Job drawing, mm, ordinate dimensions from the low corner. One solid piece. A direction names the side the tool comes from. Round coordinates to 2 decimals unless told otherwise and drop trailing zeros. Order: outer loops, then holes, each group sorted by start corner. A loop starts at its lowest first (then second) coordinate and runs counter-clockwise, first axis right, second up. Notation, with made-up numbers: (58.25, -4) - (83.25, -4) arc R10 ccw to (83.25, 1) - close; hole circle Ø9 at (-37.75, 28.5). An arc over 180 degrees is marked (long way). Write each question's results on one line, items separated by ' | '. Start each with the question number.
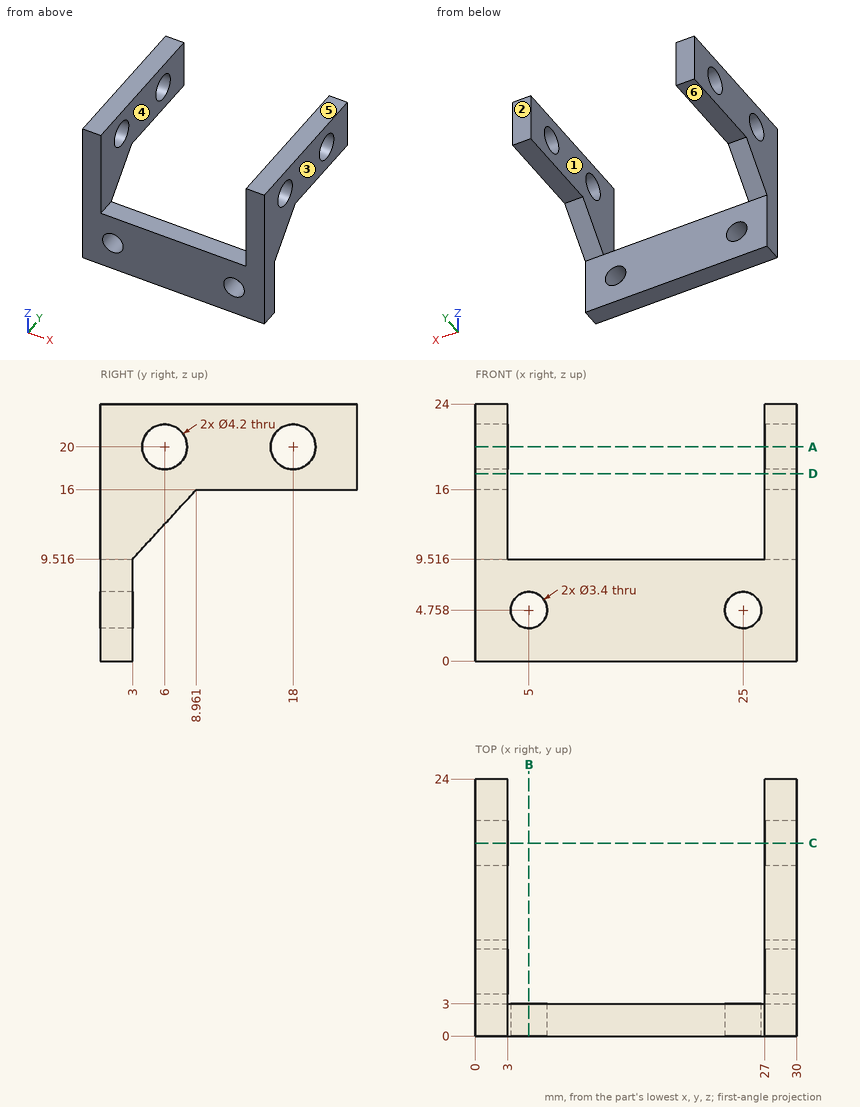
1. 3-axis set-ups, long thin cutter, end or side, ignore diameter. For the marked faces 4, 5 and 6: which of +Z, -Z, +X, -X, +Y, -Y reach the whole face in a straight line?
2. Mould opens along X. For the marked faces 1, 2 and 3 say: pulls with the +X half, pulls with the -X half, needs draft (parallel to the pull), parting line crosses it, or undercut.
3. Cut at A-A (z = 20). List the corners of the cut face in (x, y), plus the area to 3 significant figures.
4. Cut at B-B (x = 5). List the corners of the cut face in (y, z).
5. Cut at D-D (z = 17.5). List the corners of the cut face in (x, y), plus the area to 3 significant figures.
6. Flat gauge pins, fed straight in: pin 1 Ø0.9 at (x, y) = (28, 19.5) entering from -Z; pin 2 Ø3 at (x, z) = (8, 6) entering from +Y; pin 3 Ø2.5 at (x, y) = (17.5, 2) entering from +Z. Where does each tip first touch, or does it go through?
7. Cut at C-C (y = 18). List the corners of the cut face in (x, z).
8. Wall check: line 1 (Y direction, x = 27.95, z = 20); line 2 (X direction, y = 4.25, z = 14); line 3 (Z direction, x = 25, y = 1.1). Give the ranges that are in metal, low to high. Write a range as from..to.
A:
1) face 4: +Z, +Y, -Y | face 5: +Z, +X, -X, +Y, -Y | face 6: -Z, +X, -X, +Y
2) face 1: undercut | face 2: needs draft | face 3: pulls with the +X half
3) outline: (0, 0) - (3, 0) - (3, 3.9) - (0, 3.9) - close; (0, 8.1) - (3, 8.1) - (3, 15.9) - (0, 15.9) - close; (0, 20.1) - (3, 20.1) - (3, 24) - (0, 24) - close; (27, 0) - (30, 0) - (30, 3.9) - (27, 3.9) - close; (27, 8.1) - (30, 8.1) - (30, 15.9) - (27, 15.9) - close; (27, 20.1) - (30, 20.1) - (30, 24) - (27, 24) - close | area: 93.6 mm^2
4) outline: (0, 0) - (3, 0) - (3, 3.06) - (0, 3.06) - close; (0, 6.46) - (3, 6.46) - (3, 9.52) - (0, 9.52) - close
5) outline: (0, 0) - (3, 0) - (3, 24) - (0, 24) - close; (27, 0) - (30, 0) - (30, 24) - (27, 24) - close | area: 144 mm^2
6) pin 1: stops at z = 16 | pin 2: stops at y = 3 | pin 3: stops at z = 9.52
7) outline: (0, 16) - (3, 16) - (3, 17.9) - (0, 17.9) - close; (0, 22.1) - (3, 22.1) - (3, 24) - (0, 24) - close; (27, 16) - (30, 16) - (30, 17.9) - (27, 17.9) - close; (27, 22.1) - (30, 22.1) - (30, 24) - (27, 24) - close
8) line 1: y = 0..3.9, 8.1..15.9, 20.1..24 | line 2: x = 0..3, 27..30 | line 3: z = 0..3.06, 6.46..9.52
